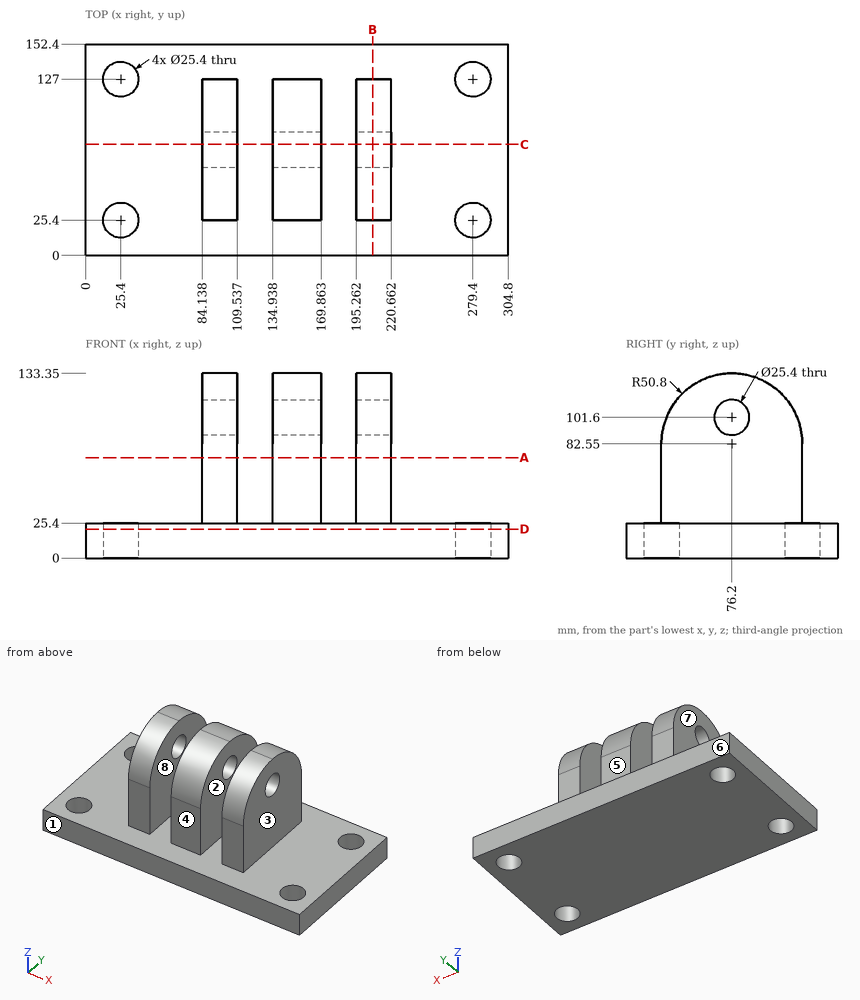
Can you work these out from the drawing? Everything is in mm from the part's minimum corner. A direction names the side the tool comes from. Coordinates: 2 decimals unless noted, no trailing zeros. Loops run counter-clockwise (first coordinate to the right, second up) from the corner with the lowest first, then second, coordinate; pieces in that order, holes last.
1) Imagine slicing it at D-D on z = 21. List the corners of the cut face in (x, y) for me.
2) Thinking about a two-plate mould opening in X: for the marked faces 1, 2 and 3, which applies, pulls with the +X half, pulls with the -X half, needs draft (parallel to the pull), parting line crosses it, or undercut?
3) I need wall thicknesses on probe 1 along Y at (x, z) = (25.4, 6.5); probe 2 along X at (y, z) = (90, 111.5); probe 3 along Z at (x, y) = (107.5, 75.5) (1 decimal). Which ranges of each line are inside material? Lowest first, please.
4) Imagine slicing it at A-A on z = 72.5. List the corners of the cut face in (x, y) for me.
5) Imagine slicing it at C-C on y = 80. List the corners of the cut face in (x, z) for me.
6) For pin 1 (4 mm diameter, centred on y = 46, z = 47.5, fed in from +X); pin 2 (8 mm diameter, centred on x = 133.5, z = 42.5, fed in from +Y); pin 3 (3 mm diameter, centred on x = 102.5, z = 108.5, fed in from -Y); pin 4 (1.5 mm diameter, centred on y = 78, z = 19.5, fed in from -X), each with a flat end and sliding along its axis, tell me the tip position at first contact or that it passes through.
7) Which directions (+Z, -Z, +X, -X, +Y, -Y) give clear straight access to the entire face, cutting with the end or side of a thin tool? Please do the marked faces 4, 5, 6, 7 and 8.
8) Imagine slicing it at B-B on x = 207. List the corners of the cut face in (y, z) for me.
Completed:
1. outline: (0, 0) - (304.8, 0) - (304.8, 152.4) - (0, 152.4) - close; hole circle Ø25.4 at (25.4, 25.4); hole circle Ø25.4 at (25.4, 127); hole circle Ø25.4 at (279.4, 25.4); hole circle Ø25.4 at (279.4, 127)
2. face 1: needs draft
2. face 2: undercut
2. face 3: pulls with the +X half
3. probe 1: y = 0 to 12.7, 38.1 to 114.3, 139.7 to 152.4
3. probe 2: x = 84.14 to 109.54, 134.94 to 169.86, 195.26 to 220.66
3. probe 3: z = 0 to 88.9, 114.3 to 133.3
4. outline: (84.14, 25.4) - (109.54, 25.4) - (109.54, 127) - (84.14, 127) - close; (134.94, 25.4) - (169.86, 25.4) - (169.86, 127) - (134.94, 127) - close; (195.26, 25.4) - (220.66, 25.4) - (220.66, 127) - (195.26, 127) - close
5. outline: (0, 0) - (304.8, 0) - (304.8, 25.4) - (220.66, 25.4) - (220.66, 89.48) - (195.26, 89.48) - (195.26, 25.4) - (169.86, 25.4) - (169.86, 89.48) - (134.94, 89.48) - (134.94, 25.4) - (109.54, 25.4) - (109.54, 89.48) - (84.14, 89.48) - (84.14, 25.4) - (0, 25.4) - close; (84.14, 113.72) - (109.54, 113.72) - (109.54, 133.21) - (84.14, 133.21) - close; (134.94, 113.72) - (169.86, 113.72) - (169.86, 133.21) - (134.94, 133.21) - close; (195.26, 113.72) - (220.66, 113.72) - (220.66, 133.21) - (195.26, 133.21) - close
6. pin 1: stops at x = 220.66
6. pin 2: stops at y = 127
6. pin 3: stops at y = 31.67
6. pin 4: stops at x = 0
7. face 4: +Z, +X, -X, -Y
7. face 5: +Z, +X, -X, +Y
7. face 6: +Z, -Z, +X, -X, +Y
7. face 7: +Z, -X, +Y, -Y
7. face 8: +Z, +Y, -Y
8. outline: (0, 0) - (152.4, 0) - (152.4, 25.4) - (127, 25.4) - (127, 82.55) arc R50.8 ccw to (25.4, 82.55) - (25.4, 25.4) - (0, 25.4) - close; hole circle Ø25.4 at (76.2, 101.6)
